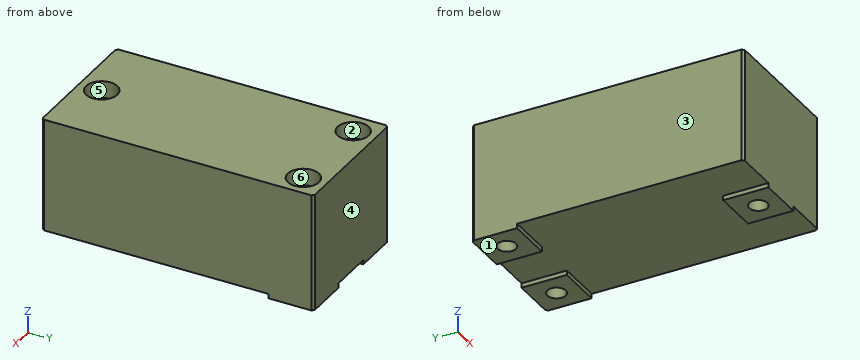
from build123d import *

# Parameters (mm, degrees)
SKETCH1_W                                        = 76.2
SKETCH1_H                                        = 152.4
EXTRUDE1_DEPTH                                   = 63.5
SKETCH4_W                                        = 25.4
SKETCH4_H                                        = 25.4
EXTRUDE2_DEPTH                                   = 2.54
CBORE_FOR_3_8_SOCKET_HEAD_CAP_SCREW1_D           = 10.31748
CBORE_FOR_3_8_SOCKET_HEAD_CAP_SCREW1_CBORE_D     = 17.4752
CBORE_FOR_3_8_SOCKET_HEAD_CAP_SCREW1_CBORE_DEPTH = 9.525
CHAMFER2_SIZE                                    = 1.27


with BuildPart() as part:
    # Sketch1 → Extrude1 (new body)
    with BuildSketch(Plane.XY):
        with Locations((0, -38.1)):
            Rectangle(SKETCH1_W, SKETCH1_H)
    extrude(amount=EXTRUDE1_DEPTH)

    # Sketch4 → Extrude2 (add)
    with BuildSketch(Plane(origin=(0, 0, 0), x_dir=(-1, 0, 0), z_dir=(0, 0, -1))):
        with Locations((-25.4, 25.4)):
            Rectangle(SKETCH4_W, SKETCH4_H)
        with Locations((25.4, 25.4)):
            Rectangle(SKETCH4_W, SKETCH4_H)
        with Locations((0, -101.6)):
            Rectangle(SKETCH4_W, SKETCH4_H)
    extrude(amount=EXTRUDE2_DEPTH)

    # CBORE for 3/8 Socket Head Cap Screw1 (through all)
    with Locations(Plane.XY.offset(63.5)):
        with Locations((-25.4, 25.4), (25.4, 25.4), (0, -101.6)):
            CounterBoreHole(CBORE_FOR_3_8_SOCKET_HEAD_CAP_SCREW1_D / 2, CBORE_FOR_3_8_SOCKET_HEAD_CAP_SCREW1_CBORE_D / 2, CBORE_FOR_3_8_SOCKET_HEAD_CAP_SCREW1_CBORE_DEPTH)

    # Chamfer2
    chamfer2_edges = [part.edges().sort_by_distance(p)[0] for p in [
        (-38.1, 38.1, 30.48),
        (38.1, 38.1, 30.48),
        (38.1, -114.3, 31.75),
        (-38.1, -114.3, 31.75),
    ]]
    chamfer(chamfer2_edges, length=CHAMFER2_SIZE)


solid = part.part
The listing builds one solid part. Answer for the finished solid, in the listing's coordinates (mm). Face numbers are marked on the shaded views. A direction names the side the tool comes from. Give positions to 0.01 mm unless a question says otherwise; leave off trailing zeros. Order: outer loops, then holes, each group sorted by start corner. A loop starts at its lowest first (then second) coordinate and runs counter-clockwise, first axis right, second up. Notation, with made-up numbers: (23.5, -6) - (57.5, -6) arc R21 ccw to (57.5, 29) - close; hole circle Ø11 at (72.25, 80.5). An arc over 180 degrees is marked (long way). One line per item, written item: value. Start each with the question number.
1) A tool of negligible diameter and unlimited length cuts with its end or side. For the marked faces 1 and 2, from which of +Z, -Z, +X, -X, +Y, -Y can it reach the whole face along a straight path? Write none if from no direction.
2) A cutting plane is placed at A-A on y = -101.6. Give the vertices of the cut face in (x, z) (3 decimals), then the cut area to 3 significant figures.
3) The mould has two halves that part along X. Classify the marked faces 3, 4, 5 and 6: released by +X, released by -X, zero draft, split by the parting line, or undercut.
4) A cutting plane is placed at B-B on x = 0. Give the vertices of the cut face in (y, z) (3 decimals), then the cut area to 3 significant figures.
5) A cutting plane is placed at D-D on y = 25.4. Give the vertices of the cut face in (x, z) (3 decimals).
6) Given pin 1 Ø1.5 at (x, y) = (1, -20.5) entering from -Z; pin 2 Ø0.8 at (y, z) = (-106.5, -1.5) entering from +X; pin 3 Ø8.5 at (x, y) = (28, 26.5) entering from +Z (3 decimals), each flat-ended and moving along its own axis, determine where each tip first touches the part or whether it passes through.
7) A cutting plane is placed at C-C on z = 41. Give the vertices of the cut face in (x, y).
8) Find the intervals of material crossed by L1, parallel to X at y = 25, z = 58; L2, parallel to Y at x = 25.4, z = 14; L3, parallel to X at y = -101, z = 61, in increasing order.
Answer sheet:
1. face 1: -Z, +X, -X, +Y, -Y
1. face 2: +Z
2. outline: (-38.1, 0) - (-12.7, 0) - (-12.7, -2.54) - (-5.159, -2.54) - (-5.159, 53.975) - (-8.738, 53.975) - (-8.738, 63.5) - (-38.1, 63.5) - close; (5.159, -2.54) - (12.7, -2.54) - (12.7, 0) - (38.1, 0) - (38.1, 63.5) - (8.738, 63.5) - (8.738, 53.975) - (5.159, 53.975) - close
2. area: 4,150 mm2
3. face 3: released by -X
3. face 4: zero draft
3. face 5: undercut
3. face 6: undercut
4. outline: (-114.3, -2.54) - (-106.759, -2.54) - (-106.759, 53.975) - (-110.338, 53.975) - (-110.338, 63.5) - (-114.3, 63.5) - close; (-96.441, -2.54) - (-88.9, -2.54) - (-88.9, 0) - (38.1, 0) - (38.1, 63.5) - (-92.862, 63.5) - (-92.862, 53.975) - (-96.441, 53.975) - close
4. area: 8,990 mm2
5. outline: (-38.1, -2.54) - (-30.559, -2.54) - (-30.559, 53.975) - (-34.138, 53.975) - (-34.138, 63.5) - (-38.1, 63.5) - close; (-20.241, -2.54) - (-12.7, -2.54) - (-12.7, 0) - (12.7, 0) - (12.7, -2.54) - (20.241, -2.54) - (20.241, 53.975) - (16.662, 53.975) - (16.662, 63.5) - (-16.662, 63.5) - (-16.662, 53.975) - (-20.241, 53.975) - close; (30.559, -2.54) - (38.1, -2.54) - (38.1, 63.5) - (34.138, 63.5) - (34.138, 53.975) - (30.559, 53.975) - close
6. pin 1: stops at z = 0
6. pin 2: stops at x = 12.7
6. pin 3: stops at z = 53.975
7. outline: (-38.1, -113.03) - (-36.83, -114.3) - (36.83, -114.3) - (38.1, -113.03) - (38.1, 36.83) - (36.83, 38.1) - (-36.83, 38.1) - (-38.1, 36.83) - close; hole circle Ø10.32 at (-25.4, 25.4); hole circle Ø10.32 at (0, -101.6); hole circle Ø10.32 at (25.4, 25.4)
8. L1: x = -38.1 to -34.13, -16.67 to 16.67, 34.13 to 38.1
8. L2: y = -114.3 to 20.24, 30.56 to 38.1
8. L3: x = -38.1 to -8.72, 8.72 to 38.1
